Work out the finished part from the listing and answer in its coordinate system (mm). Round coordinates to 2 decimals unless told otherwise and drop trailing zeros. Write each loop counter-clockwise with the first axis right and the second up, starting at its lowest first coordinate (ties: lowest second). Pieces come first, ordered by that corner, then holes. Notation, with made-up numbers: M -31,73.25 L 27,73.25 A14 cw 27,77.25 Z; hole C 31.25,-36.5 d9. An arc over 180 degrees is marked long. One line per item, written item: value. Start each with the question number.
Q1. Consider probe 1 along X at (y, z) = (-2.8, 9); probe 2 along Y at (x, z) = (-9, 1); probe 3 along X at (y, z) = (-3.7, 7). Determine where each line is inside the solid, lowest interval first.
Q2. The mould has two halves that part along X. Classify faces 1 (the cylindrical face through (-10.905, -1.061, 0.311)), 2 (the cylindrical face through (-10.862, -2.783, 0.311)), 3 (the flat face through (1, -5.08, 0)): released by +X, released by -X, zero draft, split by the parting line, or undercut.
Q3. Given pin 1 Ø1.5 at (y, z) = (-4.5, 13) entering from -X, flat-ended and moving along its own axis, determine where the tip first touches the part or whether it passes through.
Q4. Find section A-A (z = 18.5). Write down the section's boundary in (x, y).
from build123d import *

# Parameters (mm, degrees)
F1_START      = 0.508
F0_W          = 22.86
F0_H          = 44.45
F1_DEPTH      = 4.572
F2_R          = 1.397
F3_DEPTH      = 25.4
F3_DEPTH_BACK = 25.4
F4_R          = 1.8396307345
F5_R          = 1.8396307345


with BuildPart() as f1:
    # F0 (on Front) → F1 (new body)
    with BuildSketch(Plane.XZ.offset(F1_START)):
        Rectangle(F0_W, F0_H)
    extrude(amount=F1_DEPTH)

    # F2 (on Top) → F3 (cut, two sides)
    with BuildSketch(Plane.XY) as f3_sk:
        with Locations((-9.4667607918, -2.8446267825)):
            Circle(F2_R)
    extrude(amount=F3_DEPTH, mode=Mode.SUBTRACT)
    extrude(f3_sk.sketch, amount=-F3_DEPTH_BACK, mode=Mode.SUBTRACT)

    # F4
    f4_edges = [f1.edges().sort_by_distance(p)[0] for p in [
        (-11.43, -0.508, 0),
    ]]
    fillet(f4_edges, radius=F4_R)

    # F5
    f5_edges = [f1.edges().sort_by_distance(p)[0] for p in [
        (-11.43, -5.08, 0),
    ]]
    fillet(f5_edges, radius=F5_R)


solid = f1.part
The answers:
1. probe 1: -11.43 to -10.86, -8.07 to 11.43
1. probe 2: -5.08 to -4.16, -1.53 to -0.51
1. probe 3: -11.37 to -10.57, -8.36 to 11.43
2. face 1: released by -X
2. face 2: undercut
2. face 3: zero draft
3. pin 1: x = -11.36
4. outline: M -11.43,-3.24 A1.84 ccw -9.59,-5.08 L 11.43,-5.08 L 11.43,-0.51 L -9.59,-0.51 A1.84 ccw -11.43,-2.35 Z; hole C -9.47,-2.84 d2.79
